The model under review builds one solid part; all positions refer to its coordinate system, in mm. Face numbers are marked on the shaded views. A direction names the side the tool comes from. Coordinates: 2 decimals unless noted, no trailing zeros. Loops run counter-clockwise (first coordinate to the right, second up) from the corner with the lowest first, then second, coordinate; pieces in that order, holes last. Notation, with made-up numbers: M 2,-15 L 47,-15 A19 ccw 47,11 Z; hole C 56.25,3 d7. An arc over 180 degrees is marked long. One line per item, written item: value.
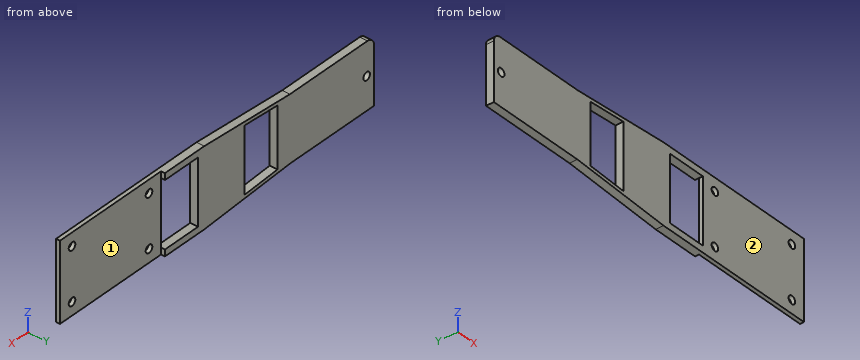
Autodesk Inventor part; units mm, degrees
ref_plane "YZ Plane" through (0, 0, 0) normal (1, 0, 0) x (0, 1, 0)
ref_plane "XZ Plane" through (0, 0, 0) normal (0, 1, 0) x (-1, 0, 0)
ref_plane "XY Plane" through (0, 0, 0) normal (0, 0, 1) x (1, 0, 0)
sketch "Sketch1" plane through (0, 0, 0) normal (0, 1, 0) x (-1, 0, 0)
  line L0 (-79.8192, 12.5065) -> (-40.859, 15)
  line L1 (-40.859, 15) -> (0, 15)
  line L2 (-80.022, 0) -> (80.022, 0) construction
  line L3 (-80.022, -12.4935) -> (-40.859, -15)
  line L4 (-40.859, -15) -> (0, -15)
  line L5 (0, 15) -> (0, -15) construction
  line L6 (40.859, 15) -> (0, 15)
  line L7 (79.8192, 12.5065) -> (40.859, 15)
  line L8 (80.022, -12.4935) -> (40.859, -15)
  line L9 (40.859, -15) -> (0, -15)
  line L10 (-59.1282, -12.5) -> (-74.1282, -11.54)
  line L11 (-59.1282, 12.5) -> (-74.1282, 11.54)
  line L12 (-74.1282, 11.54) -> (-74.1282, -11.54)
  line L13 (-59.1282, 12.5) -> (-59.1282, -12.5)
  line L14 (-23, 12.5) -> (-38, 12.5)
  line L15 (-38, 12.5) -> (-38, -12.5)
  line L16 (-38, -12.5) -> (-23, -12.5)
  line L17 (-23, -12.5) -> (-23, 12.5)
  line L18 (59.1282, -12.5) -> (74.1282, -11.54)
  line L19 (59.1282, 12.5) -> (74.1282, 11.54)
  line L20 (74.1282, 11.54) -> (74.1282, -11.54)
  line L21 (59.1282, 12.5) -> (59.1282, -12.5)
  line L22 (23, 12.5) -> (38, 12.5)
  line L23 (38, 12.5) -> (38, -12.5)
  line L24 (38, -12.5) -> (23, -12.5)
  line L25 (23, -12.5) -> (23, 12.5)
  circle A0 centre (-17.5, -10) radius 1.5
  circle A1 centre (17.5, -10) radius 1.5
  circle A2 centre (-17.5, 10) radius 1.5
  circle A3 centre (17.5, 10) radius 1.5
  line L26 (-79.8192, 12.5065) -> (-118.022, 12.5065)
  line L27 (-118.022, 12.5065) -> (-118.022, -12.4935)
  line L28 (-80.022, -12.4935) -> (-118.022, -12.4935)
  circle A4 centre (-114.702, 0) radius 1.5
  line L29 (79.8192, 12.5065) -> (118.022, 12.5065)
  line L30 (118.022, 12.5065) -> (118.022, -12.4935)
  line L31 (80.022, -12.4935) -> (118.022, -12.4935)
  circle A5 centre (114.702, 0) radius 1.5
  point P0 (0, 0)
  point P1 (0, 0)
  point P2 (0, 0)
  point P3 (-74.1282, 0)
  point P4 (-30.5, 12.5)
  dimension "d11" = 15
  dimension "d13" = 3
  dimension "d14" = 5
  dimension "d15" = 5.5
  dimension "d17" = 38
  dimension "d23" = 3
  dimension "d24" = 3.32
  dimension "d33" = 23
  dimension "d44" = 40.859
  dimension "d45" = 39.163
  dimension "d49" = 30
  dimension "d50" = 25
  dimension "d51" = 5.8938
  dimension "d52" = 15
  dimension "d53" = 25
  dimension "d54" = 1.328
extrude "Extrusion1" add sketch "Sketch1" along normal mid plane 3
fillet "Fillet1" radius 3 2 edges at (-118.022, 0, 12.5065) (118.022, 0, 12.5065)
sketch "Sketch3" plane through (-40.859, 1.5, 15) normal (0, 0, 1) x (1, 0, 0)
  line L0 (0, 0) -> (81.718, 0)
  line L1 (81.718, -3) -> (0, -3)
  line L2 (17.859, -3) -> (17.859, 0)
  line L3 (63.859, -3) -> (63.859, 0)
  line L4 (17.859, -3) -> (17.859, 0)
  line L5 (17.859, -1.5) -> (63.859, -1.5)
  line L6 (158.881, -3) -> (158.881, 0)
  line L7 (120.6782, 0) -> (155.881, 0)
  line L8 (155.881, 0) -> (158.881, 0)
  line L9 (158.881, -3) -> (155.881, -3)
  line L10 (155.881, -3) -> (120.6782, -3)
  line L11 (120.6782, -3) -> (81.718, -3)
  line L12 (81.718, 0) -> (120.6782, 0)
  line L13 (-38.9602, 0) -> (0, 0)
  line L14 (0, -3) -> (-38.9602, -3)
  line L15 (-74.163, 0) -> (-38.9602, 0)
  line L16 (-38.9602, -3) -> (-74.163, -3)
  line L17 (-77.163, 0) -> (-77.163, -3)
  line L18 (-74.163, -3) -> (-77.163, -3)
  line L19 (-77.163, 0) -> (-74.163, 0)
  point P0 (40.859, -1.5)
  point P1 (17.859, -1.5)
extrude "Extrusion3" cut sketch "Sketch3" against normal through all contours L0 L3 L5 L2 | L0 L12 L7 L8 L6 L9 L10 L11 L1 L3
properties part number "nakladka_boczna1" material "PCTG 20%"
(1) Add section D-D on y = -0.8. State the section outline as (x, z) points.
Checks:
outline: M -118.02,-12.49 L -80.02,-12.49 L -40.86,-15 L 23,-15 L 23,15 L -40.86,15 L -79.82,12.51 L -115.02,12.51 A3 ccw -118.02,9.51 Z; hole C -114.7,0 d3; hole M -74.13,-11.54 L -59.13,-12.5 L -59.13,12.5 L -74.13,11.54 Z; hole M -38,-12.5 L -23,-12.5 L -23,12.5 L -38,12.5 Z; hole C -17.5,-10 d3; hole C -17.5,10 d3; hole C 17.5,-10 d3; hole C 17.5,10 d3
(2) To check wall thickness, follow L1, parallel to X at y = -1.1, z = 5; L2, parallel to X at y = -0.85, z = -10; L3, parallel to Z at x = 17.5, y = -0.4. State the ranges of each line that lie inside material, in increasing order. Write a range as [from, to].
Checks:
L1: [-118.02, -74.13], [-59.13, -38], [-23, 23]
L2: [-118.02, -74.13], [-59.13, -38], [-23, -19], [-16, 16], [19, 23]
L3: [-15, -11.5], [-8.5, 8.5], [11.5, 15]
(3) Insertion check: pin 1 Ø1.5 at (x, y) = (-71, -0.5) entering from +Z; pin 2 Ø0.8 at (y, z) = (0.5, 14) entering from +X. Each pin has a flat end and moves straight along its axis. Give the tip position at first contact, or say it passes through.
Checks:
pin 1: z = 13.12
pin 2: x = -23
(4) Add section A-A on z = 0. State the section outline as (x, y) points.
Checks:
outline: M -118.02,-1.5 L -116.2,-1.5 L -116.2,1.5 L -118.02,1.5 Z; M -113.2,-1.5 L -74.13,-1.5 L -74.13,1.5 L -113.2,1.5 Z; M -59.13,-1.5 L -38,-1.5 L -38,1.5 L -59.13,1.5 Z; M -23,-1.5 L 23,-1.5 L 23,0 L -23,0 Z
(5) Tool access review of the marked faces 1 and 2: name each direction out of +Z, -Z, +X, -X, +Y, -Y from which nothing blocks a thin tool from reaching the whole face with its end or side.
Checks:
face 1: +Z, -Z, +X, +Y
face 2: +Z, -Z, +X, -X, -Y
(6) Add section B-B on x = -35. State the section outline as (y, z) points.
Checks:
outline: M -1.5,-15 L 1.5,-15 L 1.5,-12.5 L -1.5,-12.5 Z; M -1.5,12.5 L 1.5,12.5 L 1.5,15 L -1.5,15 Z
(7) Add section C-C on x = -17.5. State the section outline as (y, z) points.
Checks:
outline: M -1.5,-15 L 0,-15 L 0,-11.5 L -1.5,-11.5 Z; M -1.5,-8.5 L 0,-8.5 L 0,8.5 L -1.5,8.5 Z; M -1.5,11.5 L 0,11.5 L 0,15 L -1.5,15 Z
